Geometry check sheet. Reference: the model listing, model coordinates, mm. Give positions to 0.01 mm unless a question says otherwise; leave off trailing zeros. Write each loop counter-clockwise with the first axis right and the second up, starting at its lowest first coordinate (ties: lowest second). Pieces come first, ordered by that corner, then holes. Notation, with made-up numbers: (26, -27) -> (61, -27) arc R17 cw to (61, -18) -> close; hole circle Ø3 at (-3, 6). An arc over 180 degrees is marked (long way). Write item = value, one per line. Start each with the question number.
1. Mould release check, pull along X, two halves, no side actions. Record for faces 1 (the flat face through (-1, 4, 0)), 2 (the cylindrical face through (-6.883, -221.495, 31.306)), 3 (the cylindrical face through (-1.396, -253.985, 31.306)): pulls with the +X half, pulls with the -X half, needs draft (parallel to the pull), parting line crosses it, or undercut.
2. Depth check by flat-ended pin: P1, Ø2, axis at x = 20, y = 10.5, coming from the -Z side; P2, Ø5, axis at x = -50, z = 29.5, coming from the -Y side; P3, Ø4, axis at x = 40, z = 51, coming from the +Y side; P4, Ø10, axis at x = 29.5, z = 32.5, coming from the +Y side. Enter the tip coordinate at first touch or a pass-through.
3. Cross-section at D-D, the plane x = 48. Record the cut outline in (y, z).
4. Cross-section at C-C, the plane x = 26. Record the cut outline in (y, z).
5. Thickness scan on line 1 along Y through (x, z) = (0, 48); line 2 along X through (y, z) = (190, 31); line 3 along X through (y, z) = (178, 23). Record the ranges inside material, lowest first.
6. Cross-section at A-A, the plane x = 0. Record the cut outline in (y, z).
7. Cross-section at B-B, the plane z = 26.5. Record the cut outline in (x, y), plus the area to 3 significant figures.
```python
from build123d import *

# Parameters (mm, degrees)
F1_DEPTH = 63.5
F2_R     = 31.75
F3_DEPTH = 63.5


with BuildPart() as f1:
    # F0 (on Top) → F1 (new body)
    with BuildSketch(Plane.XY):
        with BuildLine():
            ThreePointArc((-63.5, -190.5), (0, -254), (63.5, -190.5))
            Line((63.5, -190.5), (-63.5, -190.5))
        make_face()
        with BuildLine():
            ThreePointArc((-63.5, -190.5), (0, -127), (63.5, -190.5))
            Line((63.5, -190.5), (63.5, 190.5))
            ThreePointArc((63.5, 190.5), (0, 127), (-63.5, 190.5))
            Line((-63.5, 190.5), (-63.5, -190.5))
        make_face()
        with BuildLine():
            Line((-63.5, -190.5), (63.5, -190.5))
            ThreePointArc((63.5, -190.5), (0, -127), (-63.5, -190.5))
        make_face()
        with BuildLine():
            ThreePointArc((-63.5, 190.5), (0, 127), (63.5, 190.5))
            Line((63.5, 190.5), (-63.5, 190.5))
        make_face()
        with BuildLine():
            Line((-63.5, 190.5), (63.5, 190.5))
            ThreePointArc((63.5, 190.5), (0, 254), (-63.5, 190.5))
        make_face()
    extrude(amount=F1_DEPTH)

    # F2 (on Top) → F3 (cut, through all)
    with BuildSketch(Plane.XY):
        with Locations((0, 190.5)):
            Circle(F2_R)
        with Locations((0, -190.5)):
            Circle(F2_R)
    extrude(amount=F3_DEPTH, mode=Mode.SUBTRACT)


solid = f1.part
```
Answers:
q1.face_1 = needs draft
q1.face_2 = undercut
q1.face_3 = parting line crosses it
q2.P1 = 0
q2.P2 = -232.64
q2.P3 = 241.37
q2.P4 = 249.08
q3.outline = (-232.07, 0) -> (232.07, 0) -> (232.07, 63.5) -> (-232.07, 63.5) -> close
q4.outline = (-248.43, 0) -> (-208.72, 0) -> (-208.72, 63.5) -> (-248.43, 63.5) -> close; (-172.28, 0) -> (172.28, 0) -> (172.28, 63.5) -> (-172.28, 63.5) -> close; (208.72, 0) -> (248.43, 0) -> (248.43, 63.5) -> (208.72, 63.5) -> close
q5.line_1 = -254 to -222.25, -158.75 to 158.75, 222.25 to 254
q5.line_2 = -63.5 to -31.75, 31.75 to 63.5
q5.line_3 = -63.5 to -29.19, 29.19 to 63.5
q6.outline = (-254, 0) -> (-222.25, 0) -> (-222.25, 63.5) -> (-254, 63.5) -> close; (-158.75, 0) -> (158.75, 0) -> (158.75, 63.5) -> (-158.75, 63.5) -> close; (222.25, 0) -> (254, 0) -> (254, 63.5) -> (222.25, 63.5) -> close
q7.outline = (-63.5, -190.5) arc R63.5 ccw to (63.5, -190.5) -> (63.5, 190.5) arc R63.5 ccw to (-63.5, 190.5) -> close; hole circle Ø63.5 at (0, -190.5); hole circle Ø63.5 at (0, 190.5)
q7.area = 54,700 mm^2
